```python
from build123d import *

# Parameters (mm, degrees)
BOSS_EXTRU_1_DEPTH = 45
ESQUISSE6_W        = 25
ESQUISSE6_H        = 7.5
BOSS_EXTRU_6_DEPTH = 18
ESQUISSE7_W        = 23
ESQUISSE7_H        = 25
BOSS_EXTRU_7_DEPTH = 2
ESQUISSE8_W        = 4.2
ESQUISSE8_H        = 0.9
BOSS_EXTRU_8_DEPTH = 5


with BuildPart() as part:
    # Esquisse1 → Boss.-Extru.1 (new body)
    with BuildSketch(Plane.XY):
        Polygon((-3.2, 0), (3.2, 0), (3.2, 2.6), (1.9, 3.9), (1.9, 5.2), (6.9, 5.2), (6.9, -2.3), (-6.9, -2.3), (-6.9, 5.2), (-1.9, 5.2), (-1.9, 3.9), (-3.2, 2.6), align=None)
    extrude(amount=BOSS_EXTRU_1_DEPTH)

    # Esquisse6 → Boss.-Extru.6 (add)
    with BuildSketch(Plane(origin=(6.9, 0, 0), x_dir=(0, 0, -1), z_dir=(1, 0, 0))):
        with Locations((-17.5, 1.45)):
            Rectangle(ESQUISSE6_W, ESQUISSE6_H)
    extrude(amount=BOSS_EXTRU_6_DEPTH)

    # Esquisse7 → Boss.-Extru.7 (add)
    with BuildSketch(Plane(origin=(0, 5.2, 0), x_dir=(1, 0, 0), z_dir=(0, 1, 0))):
        with Locations((13.4, -17.5)):
            Rectangle(ESQUISSE7_W, ESQUISSE7_H)
    extrude(amount=BOSS_EXTRU_7_DEPTH)

    # Esquisse8 → Boss.-Extru.8 (add)
    with BuildSketch(Plane(origin=(0, 7.2, 0), x_dir=(1, 0, 0), z_dir=(0, 1, 0))):
        with Locations((4, -29.55)):
            Rectangle(ESQUISSE8_W, ESQUISSE8_H)
        with Locations((4, -5.45)):
            Rectangle(ESQUISSE8_W, ESQUISSE8_H)
    extrude(amount=BOSS_EXTRU_8_DEPTH)


solid = part.part
```
Input: part model. Units: mm. Frame: model coordinates. A direction names the side the tool comes from. Coordinates: 2 decimals unless noted, no trailing zeros. Write each loop counter-clockwise with the first axis right and the second up, starting at its lowest first coordinate (ties: lowest second). Pieces come first, ordered by that corner, then holes. Notation, with made-up numbers: (11, 28) -> (18, 28) arc R25 cw to (18, 49) -> close; hole circle Ø6 at (25.5, 41). An arc over 180 degrees is marked (long way). Write each question's results on one line, items separated by ' | '.
Item 1: Set-up query: faces 1 (the flat face through (-4, 5.2, 22)), 2 (the flat face through (0, 0, 22)), 3 (the flat face through (4, 5.2, 2)), 4 (the flat face through (6.1, 9.7, 29.6)), 5 (the flat face through (4, 10, 29.1)). Return all of +Z, -Z, +X, -X, +Y, -Y with unobstructed straight access to the full face (end or side cutting, diameter ignored); none if empty.
Conclusion:
face 1: +Z, -Z, -X, +Y | face 2: +Z, -Z | face 3: -Z, +X, -X, +Y | face 4: +Z, -Z, +X, +Y | face 5: +X, -X, +Y
Item 2: Mould query, pull axis Y, two halves, no side actions, for faces 6 (the flat face through (-2.5, 3.3, 22.2)), 7 (the flat face through (6.1, 9.7, 5.5)), 8 (the flat face through (-3.2, 1, 22)), 9 (the flat face through (4, 12.2, 5.4)). Classes: +Y half, -Y half, draft (parallel to the pull), parting line (faces both ways), or undercut.
Conclusion:
face 6: undercut | face 7: draft | face 8: undercut | face 9: +Y half
Item 3: Section query C-C on y = -1. Return loops of the section in (x, z), plus the area to 3 significant figures.
Conclusion:
outline: (-6.9, 0) -> (6.9, 0) -> (6.9, 5) -> (24.9, 5) -> (24.9, 30) -> (6.9, 30) -> (6.9, 45) -> (-6.9, 45) -> close | area: 1,070 mm^2
Item 4: Section query B-B on z = 42.5. Return loops of the section in (x, y), plus the area to 3 significant figures.
Conclusion:
outline: (-6.9, -2.3) -> (6.9, -2.3) -> (6.9, 5.2) -> (1.9, 5.2) -> (1.9, 3.9) -> (3.2, 2.6) -> (3.2, 0) -> (-3.2, 0) -> (-3.2, 2.6) -> (-1.9, 3.9) -> (-1.9, 5.2) -> (-6.9, 5.2) -> close | area: 75.3 mm^2
Item 5: Material intervals for probe 1 along X at (y, z) = (4.5, 29); probe 2 along X at (y, z) = (5, 33.5); probe 3 along Z at (x, y) = (13, 3), sorted ascending.
Conclusion:
probe 1: x = -6.9 to -1.9, 1.9 to 24.9 | probe 2: x = -6.9 to -1.9, 1.9 to 6.9 | probe 3: z = 5 to 30
Item 6: Section query D-D on x = 4. Return loops of the section in (y, z), plus the area to 4 significant figures.
Conclusion:
outline: (-2.3, 0) -> (5.2, 0) -> (5.2, 5) -> (12.2, 5) -> (12.2, 5.9) -> (7.2, 5.9) -> (7.2, 29.1) -> (12.2, 29.1) -> (12.2, 30) -> (5.2, 30) -> (5.2, 45) -> (-2.3, 45) -> close | area: 396.5 mm^2
Item 7: Pin query (flat end, axial travel): pin 1 Ø0.7 at (y, z) = (9.5, 29.5) entering from +X; pin 2 Ø2.5 at (x, z) = (4, 1.5) entering from +Y; pin 3 Ø0.7 at (y, z) = (4.5, 30.5) entering from +X; pin 4 Ø7 at (x, y) = (9, 6.5) entering from -Z. Return the tip coordinate at first contact, or that it passes through.
Conclusion:
pin 1: stops at x = 6.1 | pin 2: stops at y = 5.2 | pin 3: stops at x = 6.9 | pin 4: stops at z = 0
Item 8: Section query A-A on y = 9.75. Return loops of the section in (x, z), plus the area to 3 significant figures.
Conclusion:
outline: (1.9, 5) -> (6.1, 5) -> (6.1, 5.9) -> (1.9, 5.9) -> close; (1.9, 29.1) -> (6.1, 29.1) -> (6.1, 30) -> (1.9, 30) -> close | area: 7.56 mm^2
